CAD build for the part. Positions are in the model's coordinates, mm. A direction names the side the tool comes from. Give positions to 0.01 mm unless a question says otherwise; leave off trailing zeros. Loops run counter-clockwise (first coordinate to the right, second up) from the corner with the lowest first, then second, coordinate; pieces in that order, holes last.
Item 1: Saw through at C-C on y = -2.25. Give the cut face in (x, z), plus the area to 3 significant figures.
Item 2: Mould opens along Z. For faces 4 (the flat face through (-45.925, 1.503, -10.941)), 5 (the flat face through (-34, 0, -6)), 6 (the flat face through (-30.105, 1.503, -8.533)), 7 (the cylindrical face through (-33.104, 5.497, -10.382)) say: released by +Z, released by -Z, zero draft, split by the parting line, or undercut.
Item 3: Drop flat-ended pins along their axis: P1, Ø5, axis at x = -40, z = -9.5, coming from the +Y side; P2, Ø6, axis at x = -39, y = -10.5, coming from the +Z side; P3, Ø3, axis at y = -3, z = -4.5, coming from the -X side; P4, Ø4, axis at x = -36, y = -5.5, coming from the +Z side. Give the stop position or say it passes through.
Item 4: Saw through at D-D on y = 6. Give the cut face in (x, z), plus the area to 3 significant figures.
Item 5: Probe probe 1 along X at (y, z) = (6, -9.75); probe 2 along X at (y, z) = (-6.5, -9.5); probe 3 along Z at (x, y) = (-37, 5.5). List the from-to ranges inside material, lowest first.
Item 6: Saw through at B-B on z = -1.75. Give the cut face in (x, y), plus the area to 3 significant figures.
Item 7: Saw through at A-A on y = 0.5. Give the cut face in (x, z), plus the area to 3 significant figures.
Item 8: Which spindle directions (+Z, -Z, +X, -X, +Y, -Y) get a long thin tool onto all of the face, cutting with end or side? Do faces 1 (the flat face through (-36, -9.474, -5)), 2 (the flat face through (-33.017, 1.503, -15.985)), 3 (the cylindrical face through (-38.294, 6.456, -3.393)). Say none if no direction does.
from build123d import *

# Parameters (mm, degrees)
BOSS_EXTRUDE1_DEPTH = 3.048
SKETCH2_R           = 7.493
BOSS_EXTRUDE2_DEPTH = 1.905
SKETCH3_R           = 6.35
BOSS_EXTRUDE3_DEPTH = 3.048
SKETCH5_R           = 4.953
BOSS_EXTRUDE4_DEPTH = 9.4742
SKETCH6_R           = 5.7531
BOSS_EXTRUDE5_DEPTH = 5.08
BOSS_EXTRUDE5_TAPER = 10
FILLET3_R           = 1.27
SKETCH9_R           = 4.6101
CUT_EXTRUDE2_DEPTH  = 56.100911289
SKETCH10_R          = 4.953
CUT_EXTRUDE3_DEPTH  = 5.08


with BuildPart() as part:
    # Sketch1 → Boss-Extrude1 (new body)
    with BuildSketch(Plane(origin=(0, 0, 0), x_dir=(1, 0, 0), z_dir=(0, 1, 0))):
        Polygon((-30.753854436, 4.024561232), (-29.437584499, 13.169073327), (-36.69882931, 18.881252578), (-45.276344058, 15.448919735), (-46.592613995, 6.30440764), (-39.331369184, 0.592228389), align=None)
    extrude(amount=BOSS_EXTRUDE1_DEPTH)

    # Sketch2 → Boss-Extrude2 (add)
    with BuildSketch(Plane(origin=(0, 3.048, 0), x_dir=(1, 0, 0), z_dir=(0, 1, 0))):
        with Locations(Location((-38.015099247, 9.736740484, 0), (0, 0, 90))):
            Circle(SKETCH2_R)
    extrude(amount=BOSS_EXTRUDE2_DEPTH)

    # Sketch3 → Boss-Extrude3 (add)
    with BuildSketch(Plane(origin=(0, 4.953, 0), x_dir=(1, 0, 0), z_dir=(0, 1, 0))):
        with Locations(Location((-38.015099247, 9.736740484, 0), (0, 0, 90))):
            Circle(SKETCH3_R)
    extrude(amount=BOSS_EXTRUDE3_DEPTH)

    # Sketch5 → Boss-Extrude4 (add)
    with BuildSketch(Plane.XZ):
        with Locations(Location((-38.015099247, -9.736740484, 0), (0, 0, 90))):
            Circle(SKETCH5_R)
    extrude(amount=BOSS_EXTRUDE4_DEPTH)

    # Sketch6 → Boss-Extrude5 (add)
    with BuildSketch(Plane.XZ.offset(9.4742)):
        with Locations((-38.015099247, -9.736740484)):
            Circle(SKETCH6_R)
    extrude(amount=BOSS_EXTRUDE5_DEPTH, taper=BOSS_EXTRUDE5_TAPER)

    # Fillet3
    # the kernel refuses this fillet: 1.27 mm, written as the material it takes off along each edge
    with BuildSketch(Plane(origin=(-38.015099247, 4.953, -9.736740484), x_dir=(0, 0, -1), z_dir=(1, 0, 0))) as fillet3_piece_1:
        with BuildLine():
            CenterArc((6.223, -1.263634045), FILLET3_R, 0, 84.260829523)
            Line((6.35, 0), (6.35254, 0.025272681))
            ThreePointArc((6.35254, 0.025272681), (6.9215, 0.0254), (7.493, 0.0254))
            Line((7.493, 0.0254), (7.5184, 0))
            Line((7.5184, 0), (7.5184, -1.263634045))
            Line((7.5184, -1.263634045), (7.493, -1.263634045))
        make_face()
    revolve(axis=Axis((-38.015099247, 4.953, -9.736740484), (0, 1, 0)), mode=Mode.SUBTRACT)

    # Sketch9 → Cut-Extrude2 (cut, through all)
    with BuildSketch(Plane.XZ.offset(14.5542)):
        with Locations(Location((-38.015099247, -9.736740484, 0), (0, 0, 270))):
            Circle(SKETCH9_R)
    extrude(amount=-CUT_EXTRUDE2_DEPTH, mode=Mode.SUBTRACT)

    # Sketch10 → Cut-Extrude3 (cut)
    with BuildSketch(Plane(origin=(0, 8.001, 0), x_dir=(1, 0, 0), z_dir=(0, 1, 0))):
        with Locations(Location((-38.015099247, 9.736740484, 0), (0, 0, 270))):
            Circle(SKETCH10_R)
    extrude(amount=-CUT_EXTRUDE3_DEPTH, mode=Mode.SUBTRACT)


solid = part.part
Results below:
1. outline: circle Ø9.91 at (-38.02, -9.74); hole circle Ø9.22 at (-38.02, -9.74)
1. area: 10.3 mm2
2. face 4: released by -Z
2. face 5: zero draft
2. face 6: released by +Z
2. face 7: undercut
3. P1: passes through
3. P2: stops at z = -3.98
3. P3: stops at x = -41.27
3. P4: stops at z = -4.78
4. outline: circle Ø12.7 at (-38.02, -9.74); hole circle Ø9.91 at (-38.02, -9.74)
4. area: 49.6 mm2
5. probe 1: x = -44.37 to -42.97, -33.06 to -31.67
5. probe 2: x = -42.96 to -42.62, -33.41 to -33.07
5. probe 3: z = -16.01 to -14.58, -4.89 to -3.47
6. outline: (-40.8, 0) - (-36.44, 0) - (-36.44, 3.05) - (-40.8, 3.05) - close
6. area: 13.3 mm2
7. outline: (-46.59, -6.3) - (-45.28, -15.45) - (-36.7, -18.88) - (-29.44, -13.17) - (-30.75, -4.02) - (-39.33, -0.59) - close; hole circle Ø9.22 at (-38.02, -9.74)
7. area: 155 mm2
8. face 1: none
8. face 2: -Z, +X, +Y, -Y
8. face 3: +Y
